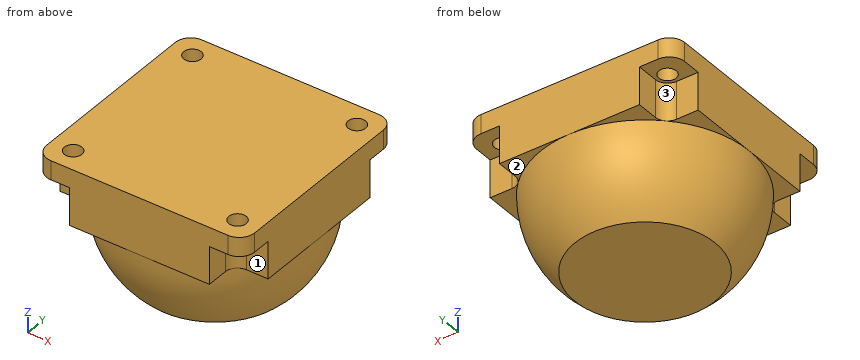
```python
from build123d import *

# Parameters (mm, degrees)
SKETCH_1_W          = 40.5
SKETCH_1_H          = 40.5
EXTRUDE_1_DEPTH     = 11
HOLE_WIZARD_M31_D   = 3.4
SKETCH_7_W          = 40.5
SKETCH_7_H          = 40.5
CUT_EXTRUDE_1_DEPTH = 11
CUT_EXTRUDE_2_DEPTH = 7.3
FILLET_1_R          = 3


with BuildPart() as part:
    # Эскиз1 → Бобышка-Вытянуть1 (new body)
    with BuildSketch(Plane.XY):
        Rectangle(SKETCH_1_W, SKETCH_1_H)
    extrude(amount=EXTRUDE_1_DEPTH)

    # Отверстие с зазором M31 (through all)
    with Locations(Plane.XY.offset(11)):
        with Locations((-16, 16), (16, 16), (16, -16), (-16, -16)):
            Hole(HOLE_WIZARD_M31_D / 2)

    # Эскиз6 → Повернуть1 (revolve)
    with BuildSketch(Plane(origin=(0, 0, 0), x_dir=(-1, 0, 0), z_dir=(0, -1, 0))):
        with BuildLine():
            Line((20.25, 0), (0, 0))
            Line((0, 0), (0, 20.25))
            ThreePointArc((0, 20.25), (14.318912319, 14.318912319), (20.25, 0))
        make_face()
    revolve(axis=Axis((0, 0, 0), (0, 0, -1)))

    # Эскиз7 → Вырез-Вытянуть1 (cut)
    with BuildSketch(Plane(origin=(0, 0, -15), x_dir=(-1, 0, 0), z_dir=(0, 0, -1))):
        Rectangle(SKETCH_7_W, SKETCH_7_H)
    extrude(amount=CUT_EXTRUDE_1_DEPTH, mode=Mode.SUBTRACT)

    # Эскиз9 → Вырез-Вытянуть2 (cut)
    with BuildSketch(Plane(origin=(0, 0, 0), x_dir=(-1, 0, 0), z_dir=(0, 0, -1))):
        with BuildLine():
            Line((-20.25, 20.25), (-13.622583002, 20.25))
            Line((-13.622583002, 20.25), (-13.622583002, 16))
            ThreePointArc((-13.622583002, 16), (-14.318912319, 14.318912319), (-16, 13.622583002))
            Line((-16, 13.622583002), (-20.25, 13.622583002))
            Line((-20.25, 13.622583002), (-20.25, 20.25))
        make_face()
        with BuildLine():
            Line((20.25, 20.25), (20.25, 13.622583002))
            Line((20.25, 13.622583002), (16, 13.622583002))
            ThreePointArc((16, 13.622583002), (14.318912319, 14.318912319), (13.622583002, 16))
            Line((13.622583002, 16), (13.622583002, 20.25))
            Line((13.622583002, 20.25), (20.25, 20.25))
        make_face()
        with BuildLine():
            Line((20.25, -20.25), (13.622583002, -20.25))
            Line((13.622583002, -20.25), (13.622583002, -16))
            ThreePointArc((13.622583002, -16), (14.318912319, -14.318912319), (16, -13.622583002))
            Line((16, -13.622583002), (20.25, -13.622583002))
            Line((20.25, -13.622583002), (20.25, -20.25))
        make_face()
        with BuildLine():
            Line((-20.25, -20.25), (-20.25, -13.622583002))
            Line((-20.25, -13.622583002), (-16, -13.622583002))
            ThreePointArc((-16, -13.622583002), (-14.318912319, -14.318912319), (-13.622583002, -16))
            Line((-13.622583002, -16), (-13.622583002, -20.25))
            Line((-13.622583002, -20.25), (-20.25, -20.25))
        make_face()
    extrude(amount=-CUT_EXTRUDE_2_DEPTH, mode=Mode.SUBTRACT)

    # Скругление1
    fillet_1_edges = [part.edges().sort_by_distance(p)[0] for p in [
        (20.25, -20.25, 9.15),
        (-20.25, -20.25, 9.15),
        (-20.25, 20.25, 9.15),
        (20.25, 20.25, 9.15),
    ]]
    fillet(fillet_1_edges, radius=FILLET_1_R)


solid = part.part
```
Design review of the part built by this model. Coordinates are the model's own, in mm. Face numbers are marked on the shaded views. A direction names the side the tool comes from. Coordinates: 2 decimals unless noted, no trailing zeros. Write each loop counter-clockwise with the first axis right and the second up, starting at its lowest first coordinate (ties: lowest second). Pieces come first, ordered by that corner, then holes.
1) Insertion check: pin 1 (2 mm diameter, centred on x = -18.5, y = 18, fed in from -Z); pin 2 (8 mm diameter, centred on x = 14.5, z = -5.5, fed in from +Y); pin 3 (1.3 mm diameter, centred on x = -18, z = 5, fed in from +Y). Each pin has a flat end and moves straight along its axis. Give the tip position at first contact, or say it passes through.
2) Add section D-D (z = -11). Write out the cut boundary in (x, y), plus the area to 3 significant figures.
3) Add section A-A (z = 5.5). Write out the cut boundary in (x, y).
4) Add section B-B (y = 4). Write out the cut boundary in (x, z).
5) To check wall thickness, follow L1, parallel to Y at x = 16, z = 9.8; L2, parallel to X at y = 18, z = 4.75; L3, parallel to Z at x = -15, y = 17.5. State the ranges of each line that lie inside material, in increasing order.
6) Machinability: for the marked faces 1, 2 and 3, which of the approach directions +Z, -Z, +X, -X, +Y, -Y give a long, thin tool a straight path to every point of the face, cutting with its end or side? Answer none if there is none.
Check result:
1. pin 1: stops at z = 7.3
1. pin 2: stops at y = 16.66
1. pin 3: stops at y = 13.62
2. outline: circle Ø34 at (0, 0)
2. area: 908 mm2
3. outline: (-20.25, -13.62) - (-16, -13.62) arc R2.38 cw to (-13.62, -16) - (-13.62, -20.25) - (13.62, -20.25) - (13.62, -16) arc R2.38 cw to (16, -13.62) - (20.25, -13.62) - (20.25, 13.62) - (16, 13.62) arc R2.38 cw to (13.62, 16) - (13.62, 20.25) - (-13.62, 20.25) - (-13.62, 16) arc R2.38 cw to (-16, 13.62) - (-20.25, 13.62) - close
4. outline: (-20.25, 0) - (-19.85, 0) arc R19.85 ccw to (-13, -15) - (13, -15) arc R19.85 ccw to (19.85, 0) - (20.25, 0) - (20.25, 11) - (-20.25, 11) - close
5. L1: y = -20.25 to -17.7, -14.3 to 14.3, 17.7 to 20.25
5. L2: x = -13.62 to 13.62
5. L3: z = 7.3 to 11
6. face 1: -Z, +X, -Y
6. face 2: -Z, +X, +Y
6. face 3: -Z, -X, +Y
